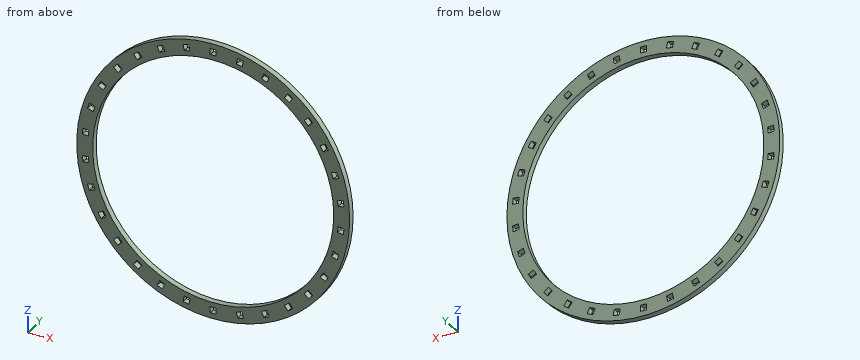
from build123d import *

# Parameters (mm, degrees)
F0_R     = 68.5
F0_R_2   = 60.5
F1_DEPTH = 3
F2_W     = 3
F2_H     = 3
F3_DEPTH = 3


with BuildPart() as f1:
    # F0 (on Front) → F1 (new body)
    with BuildSketch(Plane.XZ):
        Circle(F0_R)
        Circle(F0_R_2, mode=Mode.SUBTRACT)
    extrude(amount=F1_DEPTH)

    # F2 (on Front) → F3 (cut)
    with BuildSketch(Plane.XZ):
        with Locations((0, 64.375)):
            Rectangle(F2_W, F2_H)
        Polygon((-12.228961, 64.747341), (-15.163404, 64.123606), (-14.539669, 61.189163), (-11.605226, 61.812898), align=None)
        Polygon((-25.423458, 60.789912), (-28.164095, 59.569702), (-26.943885, 56.829066), (-24.203248, 58.049276), align=None)
        Polygon((-35.743472, 51.748621), (-37.506828, 54.175672), (-39.933879, 52.412317), (-38.170523, 49.985266), align=None)
        Polygon((-45.721535, 43.186304), (-47.950969, 45.193696), (-49.958361, 42.964261), (-47.728927, 40.95687), align=None)
        Polygon((-53.701347, 32.736538), (-56.299423, 34.236538), (-57.799423, 31.638462), (-55.201347, 30.138462), align=None)
        Polygon((-59.334153, 20.856028), (-62.187323, 21.783079), (-63.114374, 18.92991), (-60.261204, 18.002859), align=None)
        Polygon((-62.373771, 8.06401), (-65.357337, 8.377595), (-65.670923, 5.39403), (-62.687357, 5.080444), align=None)
        Polygon((-62.687357, -5.080444), (-65.670923, -5.39403), (-65.357337, -8.377595), (-62.373771, -8.06401), align=None)
        Polygon((-60.261204, -18.002859), (-63.114374, -18.92991), (-62.187323, -21.783079), (-59.334153, -20.856028), align=None)
        Polygon((-55.201347, -30.138462), (-57.799423, -31.638462), (-56.299423, -34.236538), (-53.701347, -32.736538), align=None)
        Polygon((-47.728927, -40.95687), (-49.958361, -42.964261), (-47.950969, -45.193696), (-45.721535, -43.186304), align=None)
        Polygon((-38.170523, -49.985266), (-39.933879, -52.412317), (-37.506828, -54.175672), (-35.743472, -51.748621), align=None)
        Polygon((-26.943885, -56.829066), (-28.164095, -59.569702), (-25.423458, -60.789912), (-24.203248, -58.049276), align=None)
        Polygon((-14.539669, -61.189163), (-15.163404, -64.123606), (-12.228961, -64.747341), (-11.605226, -61.812898), align=None)
        with Locations((0, -64.375)):
            Rectangle(F2_W, F2_H)
        Polygon((11.605226, -61.812898), (12.228961, -64.747341), (15.163404, -64.123606), (14.539669, -61.189163), align=None)
        Polygon((24.203248, -58.049276), (25.423458, -60.789912), (28.164095, -59.569702), (26.943885, -56.829066), align=None)
        Polygon((35.743472, -51.748621), (37.506828, -54.175672), (39.933879, -52.412317), (38.170523, -49.985266), align=None)
        Polygon((45.721535, -43.186304), (47.950969, -45.193696), (49.958361, -42.964261), (47.728927, -40.95687), align=None)
        Polygon((53.701347, -32.736538), (56.299423, -34.236538), (57.799423, -31.638462), (55.201347, -30.138462), align=None)
        Polygon((59.334153, -20.856028), (62.187323, -21.783079), (63.114374, -18.92991), (60.261204, -18.002859), align=None)
        Polygon((62.373771, -8.06401), (65.357337, -8.377595), (65.670923, -5.39403), (62.687357, -5.080444), align=None)
        Polygon((62.687357, 5.080444), (65.670923, 5.39403), (65.357337, 8.377595), (62.373771, 8.06401), align=None)
        Polygon((60.261204, 18.002859), (63.114374, 18.92991), (62.187323, 21.783079), (59.334153, 20.856028), align=None)
        Polygon((55.201347, 30.138462), (57.799423, 31.638462), (56.299423, 34.236538), (53.701347, 32.736538), align=None)
        Polygon((47.728927, 40.95687), (49.958361, 42.964261), (47.950969, 45.193696), (45.721535, 43.186304), align=None)
        Polygon((38.170523, 49.985266), (39.933879, 52.412317), (37.506828, 54.175672), (35.743472, 51.748621), align=None)
        Polygon((26.943885, 56.829066), (28.164095, 59.569702), (25.423458, 60.789912), (24.203248, 58.049276), align=None)
        Polygon((14.539669, 61.189163), (15.163404, 64.123606), (12.228961, 64.747341), (11.605226, 61.812898), align=None)
    extrude(amount=F3_DEPTH, mode=Mode.SUBTRACT)


solid = f1.part
Geometry: final body of the model. Coordinates: model frame, mm. Coordinates: 2 decimals unless noted, no trailing zeros. Write each loop counter-clockwise with the first axis right and the second up, starting at its lowest first coordinate (ties: lowest second). Pieces come first, ordered by that corner, then holes. Notation, with made-up numbers: (-22.75, -15) - (-18.75, -15) arc R17 cw to (-18.75, -4) - close; hole circle Ø10 at (-16.5, 39). An arc over 180 degrees is marked (long way). Return JSON: item names as keys, results as strings.
Item 1: Section query A-A (z = 0). Output: boundary loops of the cut face in (x, y), and give its area (3 significant figures).
Completed:
{"outline": "(-68.5, -3) - (-60.5, -3) - (-60.5, 0) - (-68.5, 0) - close; (60.5, -3) - (68.5, -3) - (68.5, 0) - (60.5, 0) - close", "area": "48.0 mm2"}
Item 2: Section query B-B (x = 20). Output: boundary loops of the cut face in (y, z), and give its area (3 significant figures).
Completed:
{"outline": "(-3, -65.52) - (0, -65.52) - (0, -57.1) - (-3, -57.1) - close; (-3, 57.1) - (0, 57.1) - (0, 65.52) - (-3, 65.52) - close", "area": "50.5 mm2"}
Item 3: Pin query (flat end, axial travel): pin 1 Ø1.5 at (x, y) = (-0.5, -1.5) entering from -Z. Return the tip coordinate at first contact, or that it passes through.
Completed:
{"pin 1": "stops at z = -68.5"}
Item 4: Line query: L1, parallel to Z at x = 0, y = -1.3 (3 decimals); L2, parallel to X at y = -1.9, z = -0.5; L3, parallel to Z at x = 39, y = -2.35. Output: solid intervals per line, ascending.
Completed:
{"L1": "z = -68.5 to -65.875, -62.875 to -60.5, 60.5 to 62.875, 65.875 to 68.5", "L2": "x = -68.5 to -60.5, 60.5 to 68.5", "L3": "z = -56.31 to -53.09, -51.13 to -46.25, 46.25 to 51.13, 53.09 to 56.31"}
Item 5: Section query C-C (y = -1). Count the separate pieces of the cut face and the enclosed holes in it, and give its area (3 significant figures).
Completed:
{"separate pieces": "1", "enclosed holes": "31", "area": "2,970 mm2"}
